Part model, mm, in its own coordinate system. A direction names the side the tool comes from. Round coordinates to 2 decimals unless told otherwise and drop trailing zeros. Loops run counter-clockwise (first coordinate to the right, second up) from the corner with the lowest first, then second, coordinate; pieces in that order, holes last. Notation, with made-up numbers: M 36,76 L 83,76 A9 cw 83,87 Z; hole C 51,-18 d7. An arc over 180 degrees is marked long. Answer as CSV lines item,"result". Start each with the question number.
Item 1: Which spindle directions (+Z, -Z, +X, -X, +Y, -Y) get a long thin tool onto all of the face, cutting with end or side? Do faces 1 (the flat face through (0, 5, -4)), 2 (the cylindrical face through (0.33, 7.46, 29.48)), 3 (the cylindrical face through (-0.59, 4.46, 9.86)). Say none if no direction does.
Item 2: Drop flat-ended pins along their axis: pin 1 Ø6 at (x, z) = (2, -2.5) entering from +Y; pin 2 Ø4 at (y, z) = (2, 11) entering from -X; pin 3 Ø1.6 at (x, z) = (-4, -9.5) entering from -Y. Give the stop position or say it passes through.
Item 3: Band-saw the part on A-A (y = 0). Give the cut face in (x, z), and give its area (4 significant figures).
Item 4: Mould opens along Z. For faces 4 (the flat face through (0, 0, 30)), 5 (the flat face through (-5, 0, -4)), 6 (the flat face through (-4, 0, 20.75)) say: pulls with the +Z half, pulls with the -Z half, needs draft (parallel to the pull), parting line crosses it, or undercut.
Item 5: Band-saw the part on D-D (z = 5). Give the cut face in (x, y).
Item 6: Wall check: line 1 (Z direction, x = -2.5, y = -4); line 2 (Z direction, x = -2, y = 3.25); line 3 (Y direction, x = 0.5, z = 24). Give the ranges that are in metal, low to high.
Item 7: Band-saw the part on C-C (z = 27). Give the cut face in (x, y), and give its area (3 significant figures).
```python
from build123d import *

# Parameters (mm, degrees)
F0_R      = 4.5
F1_DEPTH  = 20
F0_W      = 10
F0_H      = 10
F2_DEPTH  = 7
F4_W      = 10
F4_H      = 10
F5_DEPTH  = 10
F6_R      = 2.5
F7_DEPTH  = 5
F8_T      = -0.75
F9_W      = 2
F9_H      = 2
F10_DEPTH = 4


with BuildPart() as f1:
    # F0 (on Top) → F1 (new body)
    with BuildSketch(Plane.XY):
        Circle(F0_R)
    extrude(amount=F1_DEPTH)

    # F0 (on Top) → F2 (join)
    with BuildSketch(Plane.XY):
        Rectangle(F0_W, F0_H)
        Circle(F0_R, mode=Mode.SUBTRACT)
        Circle(F0_R)
    extrude(amount=-F2_DEPTH)

    # F4 (on offset) → F5 (join)
    with BuildSketch(Plane.XY.offset(20)):
        Rectangle(F4_W, F4_H)
    extrude(amount=F5_DEPTH)

    # F6 (on face) → F7 (join)
    with BuildSketch(Plane(origin=(0, 5, 0), x_dir=(-1, 0, 0), z_dir=(0, 1, 0))):
        with Locations((0, 27)):
            Circle(F6_R)
    extrude(amount=F7_DEPTH)

    # F8
    f8_openings = [f1.faces().sort_by_distance(p)[0] for p in [
        (0, 10, 27),
    ]]
    offset(amount=F8_T, openings=f8_openings, kind=Kind.INTERSECTION)

    # F9 (on face) → F10 (join)
    with BuildSketch(Plane(origin=(0, 0, -7), x_dir=(1, 0, 0), z_dir=(0, 0, -1))):
        with Locations((4, -4)):
            Rectangle(F9_W, F9_H)
        with Locations((-4, -4)):
            Rectangle(F9_W, F9_H)
    extrude(amount=F10_DEPTH)


solid = f1.part
```
Answer block:
1,face 1,"-Z, +X, -X, +Y"
1,face 2,"+Y"
1,face 3,"none"
2,pin 1,"stops at y = 5"
2,pin 2,"stops at x = -4.5"
2,pin 3,"stops at y = 3"
3,outline,"M -5,-7 L 5,-7 L 5,0 L 4.5,0 L 4.5,20 L 5,20 L 5,30 L -5,30 L -5,20 L -4.5,20 L -4.5,0 L -5,0 Z; hole M -4.25,-6.25 L 4.25,-6.25 L 4.25,-0.75 L 3.75,-0.75 L 3.75,20.75 L 4.25,20.75 L 4.25,29.25 L -4.25,29.25 L -4.25,20.75 L -3.75,20.75 L -3.75,-0.75 L -4.25,-0.75 Z"
3,area,"69.75 mm^2"
4,face 4,"pulls with the +Z half"
4,face 5,"needs draft"
4,face 6,"undercut"
5,outline,"C 0,0 d9; hole C 0,0 d7.5"
6,line 1,"z = -7 to -6.25, -0.75 to 0, 20 to 20.75, 29.25 to 30"
6,line 2,"z = -7 to -6.25, -0.75 to 20.75, 29.25 to 30"
6,line 3,"y = -5 to -4.25, 4.25 to 5"
7,outline,"M -5,-5 L 5,-5 L 5,5 L 2.5,5 L 2.5,10 L 1.75,10 L 1.75,4.25 L 4.25,4.25 L 4.25,-4.25 L -4.25,-4.25 L -4.25,4.25 L -1.75,4.25 L -1.75,10 L -2.5,10 L -2.5,5 L -5,5 Z"
7,area,"32.6 mm^2"
